```python
from build123d import *

# Parameters (mm, degrees)
SKETCH_2_R          = 2.5
EXTRUDE_1_DEPTH     = 10
SKETCH_3_R          = 2
CUT_EXTRUDE_2_DEPTH = 43


with BuildPart() as part:
    # Эскиз2 → Вытянуть1 (new body)
    with BuildSketch(Plane(origin=(0, 0, 0), x_dir=(0, 0, -1), z_dir=(1, 0, 0))):
        Polygon((0, 5), (40, 5), (40, 9), (28, 9), (28, 13.077507284), (25.234860189, 17), (14.765139811, 17), (12, 13.077507284), (12, 9), (0, 9), align=None)
        with Locations((20, 12)):
            Circle(SKETCH_2_R, mode=Mode.SUBTRACT)
    extrude(amount=EXTRUDE_1_DEPTH)

    # Эскиз3 → Вытянуть2 (cut, through all)
    with BuildSketch(Plane(origin=(0, 9, 0), x_dir=(1, 0, 0), z_dir=(0, 1, 0))):
        with Locations(Location((5, 6, 0), (0, 0, 270))):
            Circle(SKETCH_3_R)
        with Locations(Location((5, 34, 0), (0, 0, 90))):
            Circle(SKETCH_3_R)
    extrude(amount=-CUT_EXTRUDE_2_DEPTH, mode=Mode.SUBTRACT)


solid = part.part
```
Work out the finished part from the listing and answer in its coordinate system (mm). A direction names the side the tool comes from. Give positions to 0.01 mm unless a question says otherwise; leave off trailing zeros. Loops run counter-clockwise (first coordinate to the right, second up) from the corner with the lowest first, then second, coordinate; pieces in that order, holes last. Notation, with made-up numbers: (59.5, 86.25) - (67.5, 86.25) arc R24 ccw to (67.5, 117.25) - close; hole circle Ø7 at (38, 52.5). An arc over 180 degrees is marked (long way). Use CSV: the item, a comma, the result in double quotes. Start each with the question number.
(1) Find the intervals of material crossed by L1, parallel to Z at x = 3.5, y = 6; L2, parallel to X at y = 6.5, z = -6; L3, parallel to Y at x = 6.5, z = -20, in increasing order.
(2) A tool of negligible diameter and unlimited length cuts with its end or side. For faces 1 (the face through (5, 11, -28)), 2 (the face through (5, 11, -12)), 3 (the face through (5, 5, -20)), from which of +Z, -Z, +X, -X, +Y, -Y can it reach the whole face along a straight path? Write none if from no direction.
(3) Find section B-B, the plane z = -20. Determine the outline of the cut face in (x, y), plus the area to 3 significant figures.
(4) Find section C-C, the plane y = 10. Determine the outline of the cut face in (x, z).
(5) Find section D-D, the plane x = 9.25. Determine the outline of the cut face in (y, z).
(6) Each of these flat-tipped pins is pushed along its axis until it touches: pin 1 (3 mm diameter, centred on x = 5.5, z = -6.5, fed in from +Y); pin 2 (2 mm diameter, centred on x = 2.5, y = 12, fed in from -Z); pin 3 (2 mm diameter, centred on x = 2.5, y = 10.5, fed in from +Z). Where does it stop, or does it pass through?
(7) Find section A-A, the plane x = 5. Determine the outline of the cut face in (y, z), plus the area to 3 significant figures.
(8) Determine the mould class of faces 4 (the face through (4.93, 15.066, -13.402)), 5 (the face through (5.766, 7.028, -35.847)), 6 (the face through (2.7, 9, -34.1)) for opening direction Z: released by +Z, released by -Z, zero draft, split by the parting line, or undercut.
Results found:
1,L1,"-40 to -35.32, -32.68 to -7.32, -4.68 to 0"
1,L2,"0 to 3, 7 to 10"
1,L3,"5 to 9.5, 14.5 to 17"
2,face 1,"-Z, +X, -X, +Y"
2,face 2,"+Z, +X, -X, +Y"
2,face 3,"+Z, -Z, +X, -X, -Y"
3,outline,"(0, 5) - (10, 5) - (10, 9.5) - (0, 9.5) - close; (0, 14.5) - (10, 14.5) - (10, 17) - (0, 17) - close"
3,area,"70.0 mm^2"
4,outline,"(0, -28) - (10, -28) - (10, -21.5) - (0, -21.5) - close; (0, -18.5) - (10, -18.5) - (10, -12) - (0, -12) - close"
5,outline,"(5, -40) - (9, -40) - (9, -28) - (13.08, -28) - (17, -25.23) - (17, -14.77) - (13.08, -12) - (9, -12) - (9, 0) - (5, 0) - close; hole circle Ø5 at (12, -20)"
6,pin 1,"y = 9"
6,pin 2,"z = -28"
6,pin 3,"z = -12"
7,outline,"(5, -40) - (9, -40) - (9, -36) - (5, -36) - close; (5, -32) - (9, -32) - (9, -28) - (13.08, -28) - (17, -25.23) - (17, -14.77) - (13.08, -12) - (9, -12) - (9, -8) - (5, -8) - close; (5, -4) - (9, -4) - (9, 0) - (5, 0) - close; hole circle Ø5 at (12, -20)"
7,area,"226 mm^2"
8,face 4,"released by +Z"
8,face 5,"undercut"
8,face 6,"zero draft"
